Autodesk Inventor part; units mm, degrees
ref_plane "YZ Plane" through (0, 0, 0) normal (1, 0, 0) x (0, 1, 0)
ref_plane "XZ Plane" through (0, 0, 0) normal (0, 1, 0) x (-1, 0, 0)
ref_plane "XY Plane" through (0, 0, 0) normal (0, 0, 1) x (1, 0, 0)
sketch "Sketch1" plane through (0, 0, 0) normal (0, 0, 1) x (1, 0, 0)
  line L0 (-54.6, 49.4) -> (54.6, 49.4)
  line L1 (54.6, 49.4) -> (54.6, -49.4)
  line L2 (54.6, -49.4) -> (-54.6, -49.4)
  line L3 (-54.6, -49.4) -> (-54.6, 49.4)
  line L4 (-54.6, 49.4) -> (54.6, -49.4) construction
  line L5 (54.6, 49.4) -> (-54.6, -49.4) construction
  point P0 (0, 0)
  dimension "Comp" = 109.2
  dimension "Larg" = 98.8
extrude "Extrusion1" add sketch "Sketch1" along normal mid plane 6.5
hole "Hole2" at (-40.6, 0, 3.25) direction (0, 0, -1) diameter 13 end through all
hole "Hole3" at (29.25, 0, 3.25) direction (0, 0, -1) diameter 13 end through all
properties part number "Buste3-2"
Design review of the part built by this model. Coordinates are the model's own, in mm. Coordinates: 2 decimals unless noted, no trailing zeros. Order: outer loops, then holes, each group sorted by start corner. A loop starts at its lowest first (then second) coordinate and runs counter-clockwise, first axis right, second up.
1) Wall thickness on line 1 along X through (y, z) = (0, -1.5); line 2 along Y through (x, z) = (29.25, -2); line 3 along X through (y, z) = (1.5, 2): over which ranges is each line inside the solid? List them lowest first.
2) Mouldability with a two-part tool opening along X and no side actions: class faces 1 (the flat face through (54.6, 1, 0)), 2 (the flat face through (1, -49.4, 0)), 3 (the cylindrical face through (-47.045, 0.846, -0.046)) as +X half, -X half, draft (parallel to the pull), parting line (faces both ways), or undercut.
3) Clearance check with a flat-ended pin moving along its axis: pin 1 (11.5 mm diameter, centred on x = -40.6, y = 0, fed in from +Z). State where the tip first meets the part, or that it passes through.
4) Take a section at B-B, the plane x = -40.6. Give the boundary of the cut face in (y, z).
5) Take a section at A-A, the plane y = 0. Give the boundary of the cut face in (x, z), and give its area (3 significant figures).
6) Take a section at C-C, the plane z = -1.75. Give the boundary of the cut face in (x, y).
Returned:
1. line 1: x = -54.6 to -47.1, -34.1 to 22.75, 35.75 to 54.6
1. line 2: y = -49.4 to -6.5, 6.5 to 49.4
1. line 3: x = -54.6 to -46.92, -34.28 to 22.93, 35.57 to 54.6
2. face 1: +X half
2. face 2: draft
2. face 3: undercut
3. pin 1: passes through
4. outline: (-49.4, -3.25) - (-6.5, -3.25) - (-6.5, 3.25) - (-49.4, 3.25) - close; (6.5, -3.25) - (49.4, -3.25) - (49.4, 3.25) - (6.5, 3.25) - close
5. outline: (-54.6, -3.25) - (-47.1, -3.25) - (-47.1, 3.25) - (-54.6, 3.25) - close; (-34.1, -3.25) - (22.75, -3.25) - (22.75, 3.25) - (-34.1, 3.25) - close; (35.75, -3.25) - (54.6, -3.25) - (54.6, 3.25) - (35.75, 3.25) - close
5. area: 541 mm2
6. outline: (-54.6, -49.4) - (54.6, -49.4) - (54.6, 49.4) - (-54.6, 49.4) - close; hole circle Ø13 at (-40.6, 0); hole circle Ø13 at (29.25, 0)
